Source: three-view drawing plus pictorial views. Frame: mm from the lowest corner of the part. A direction names the side the tool comes from. Round coordinates to 2 decimals unless told otherwise and drop trailing zeros. Loops run counter-clockwise (first coordinate to the right, second up) from the corner with the lowest first, then second, coordinate; pieces in that order, holes last. Notation, with made-up numbers: M -40,-22 L -7,-22 A13 cw -7,-14 Z; hole C 56.25,67 d5. An arc over 180 degrees is marked long. Answer as a JSON object with one key per item and string values.
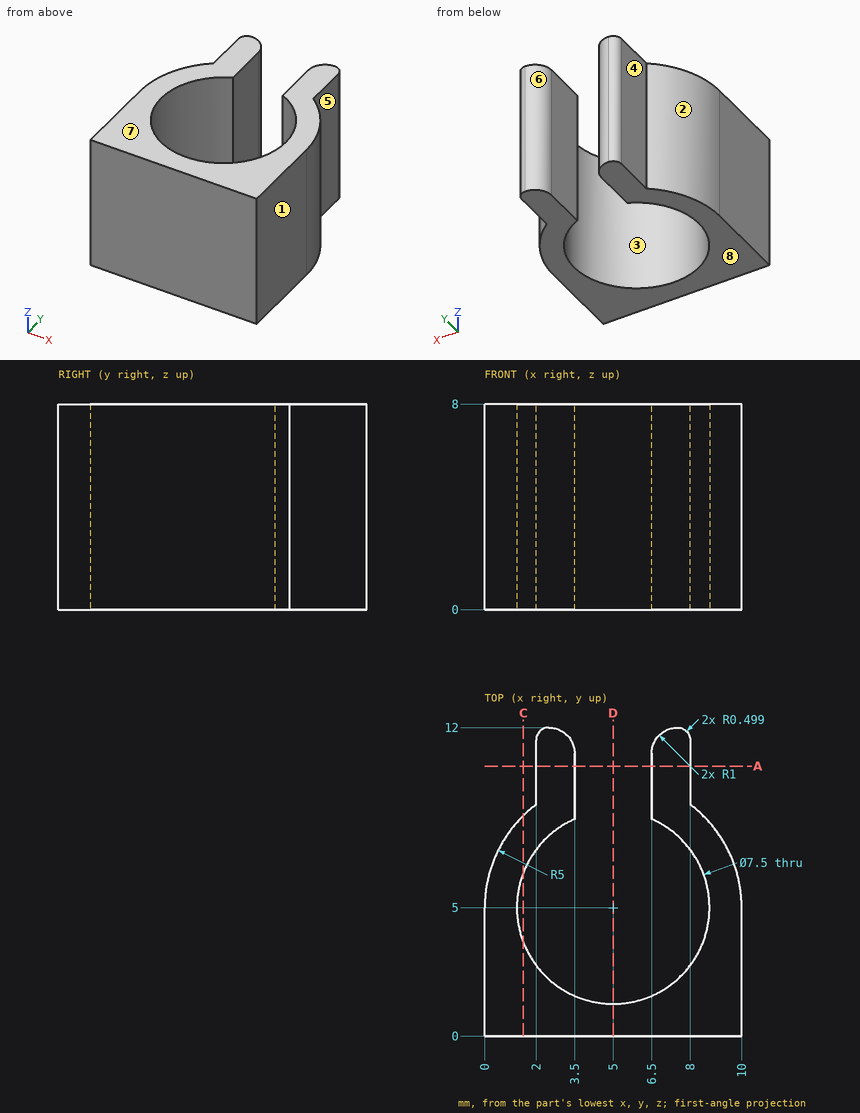
1) Cut plane D-D on x = 5. Return the cut outline in (y, z), and give its area (3 significant figures).
Geometry results:
{"outline": "M 0,0 L 1.25,0 L 1.25,8 L 0,8 Z", "area": "10.0 mm2"}
2) Cut plane C-C on x = 1.5. Return the cut outline in (y, z).
Geometry results:
{"outline": "M 0,0 L 3.65,0 L 3.65,8 L 0,8 Z; M 6.35,0 L 8.57,0 L 8.57,8 L 6.35,8 Z"}
3) Pull-direction query (X, two-part tool) for the marked faces 1, 2 and 3; classes: +X half, -X half, draft (parallel to the pull), parting line (faces both ways), or undercut.
Geometry results:
{"face 1": "+X half", "face 2": "-X half", "face 3": "undercut"}
4) Line query: probe 1 along X at (y, z) = (5, 5.75); probe 2 along X at (y, z) = (9.5, 3); probe 3 along Y at (x, z) = (5, 5.25). Output: solid intervals per line, ascending.
Geometry results:
{"probe 1": "0 to 1.25, 8.75 to 10", "probe 2": "2 to 3.5, 6.5 to 8", "probe 3": "0 to 1.25"}
5) First-contact query: pin 1 (2 mm diameter, centred on y = 6.5, z = 2, fed in from -X) (1 decimal); pin 2 (1.5 mm diameter, centred on x = 4.5, z = 2, fed in from +Y) (1 decimal); pin 3 (2 mm diameter, centred on y = 10.5, z = 2.5, fed in from +X). Flat tips, straight axial feed; report the tip coordinate or a pass-through.
Geometry results:
{"pin 1": "x = 0", "pin 2": "y = 1.5", "pin 3": "x = 8"}
6) Set-up query: the marked faces 4, 5, 6, 7 and 8. Return all of +Z, -Z, +X, -X, +Y, -Y with unobstructed straight access to the full face (end or side cutting, diameter ignored); none if empty.
Geometry results:
{"face 4": "+Z, -Z, -X, +Y", "face 5": "+Z, -Z, +X, +Y", "face 6": "+Z, -Z, +Y", "face 7": "+Z, +X, -X, +Y, -Y", "face 8": "-Z, +X, -X, +Y, -Y"}
7) Cut plane A-A on y = 10.5. Return the cut outline in (x, z).
Geometry results:
{"outline": "M 2,0 L 3.5,0 L 3.5,8 L 2,8 Z; M 6.5,0 L 8,0 L 8,8 L 6.5,8 Z"}
